Source: CAD feature listing. Evaluate the final solid. Frame: model axes, mm. Face numbers are marked on the shaded views. A direction names the side the tool comes from. Give positions to 0.01 mm unless a question says otherwise; leave off trailing zeros. Order: outer loops, then holes, each group sorted by start corner. A loop starts at its lowest first (then second) coordinate and runs counter-clockwise, first axis right, second up. Notation, with made-up numbers: (54, 66.25) - (76, 66.25) arc R14 ccw to (76, 75.25) - close; hole circle Ø7 at (-12.75, 42.5). An arc over 180 degrees is marked (long way). Answer as CSV lines item,"result".
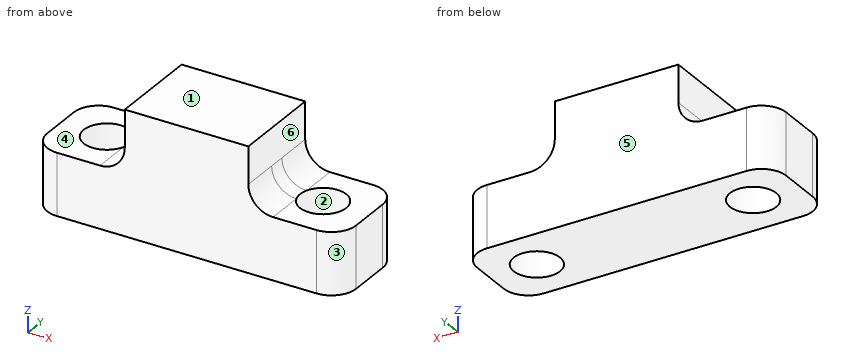
```python
from build123d import *

# Parameters (mm, degrees)
F1_DEPTH = 19.05
F3_DEPTH = 25.4
F4_R     = 5.08


with BuildPart() as f1:
    # F0 (on Front) → F1 (new body)
    with BuildSketch(Plane.XZ):
        Polygon((0, 12.7), (0, 0), (31.75, 0), (31.75, 25.4), (19.05, 25.4), (19.05, 12.7), align=None)
    extrude(amount=F1_DEPTH)

    # F2 (on face) → F3 (cut)
    with BuildSketch(Plane.XY.offset(12.7)):
        with BuildLine():
            ThreePointArc((14.2875, -9.525), (12.8925960454, -6.1574039546), (9.525, -4.7625))
            Line((9.525, -4.7625), (9.525, -9.525))
            Line((9.525, -9.525), (4.7625, -9.525))
            ThreePointArc((4.7625, -9.525), (9.525, -14.2875), (14.2875, -9.525))
        make_face()
        with BuildLine():
            Line((9.525, -9.525), (9.525, -4.7625))
            ThreePointArc((9.525, -4.7625), (6.1574039546, -6.1574039546), (4.7625, -9.525))
            Line((4.7625, -9.525), (9.525, -9.525))
        make_face()
    extrude(amount=-F3_DEPTH, mode=Mode.SUBTRACT)

    # F4
    f4_edges = [f1.edges().sort_by_distance(p)[0] for p in [
        (0, -19.05, 6.35),
        (0, 0, 6.35),
        (19.05, -9.525, 12.7),
    ]]
    fillet(f4_edges, radius=F4_R)

    # F5: F1 across face


with BuildPart() as f1_1:
    add(f1.part)
    add(f1.part.mirror(Plane(origin=(31.75, -9.525, 12.7), x_dir=(0, 1, 0), z_dir=(1, 0, 0))))


solid = f1_1.part
```
(1) Cut plane C-C (z = 6.5). Give the number of separate pieces and of enclosed holes in the cut face, then the cut area to 3 significant figures.
Completed:
separate pieces,"1"
enclosed holes,"2"
area,"1,050 mm²"
(2) Cut plane B-B (x = 51.5). Return loops of the section in (y, z), then the cut area to 3 significant figures.
Completed:
outline,"(-19.05, 0) - (-13.59, 0) - (-13.59, 12.7) - (-19.05, 12.7) - close; (-5.46, 0) - (0, 0) - (0, 12.7) - (-5.46, 12.7) - close"
area,"139 mm²"
(3) Contact query for flat-ended pins moving along their axis: pin 1 (4 mm diameter, centred on x = 5.5, y = -8.5, fed in from +Z); pin 2 (2.5 mm diameter, centred on y = -6.5, z = 23, fed in from -X); pin 3 (2.5 mm diameter, centred on y = -9, z = 19.5, fed in from +X). Output: stop coordinate, or through.
Completed:
pin 1,"z = 12.7"
pin 2,"x = 19.05"
pin 3,"x = 44.45"
(4) Mould query, pull axis Y, two halves, no side actions, for the marked faces 1, 2 and 3. Classes: released by +Y, released by -Y, zero draft, split by the parting line, or undercut.
Completed:
face 1,"zero draft"
face 2,"undercut"
face 3,"released by -Y"
(5) Cut plane D-D (y = -15.25). Return loops of the section in (x, z), then the cut area to 3 significant figures.
Completed:
outline,"(0.16, 0) - (63.34, 0) - (63.34, 12.7) - (49.53, 12.7) arc R5.08 cw to (44.45, 17.78) - (44.45, 25.4) - (19.05, 25.4) - (19.05, 17.78) arc R5.08 cw to (13.97, 12.7) - (0.16, 12.7) - close"
area,"1,140 mm²"
(6) Cut plane A-A (y = -12). Return loops of the section in (x, z).
Completed:
outline,"(0, 0) - (5.46, 0) - (5.46, 12.7) - (0, 12.7) - close; (13.59, 0) - (49.91, 0) - (49.91, 12.7) - (49.53, 12.7) arc R5.08 cw to (44.45, 17.78) - (44.45, 25.4) - (19.05, 25.4) - (19.05, 17.78) arc R5.08 cw to (13.97, 12.7) - (13.59, 12.7) - close; (58.04, 0) - (63.5, 0) - (63.5, 12.7) - (58.04, 12.7) - close"
(7) Access query for the marked faces 4, 5 and 6. Directions: +Z, -Z, +X, -X, +Y, -Y. A direction counts if a zero-diameter tool reaches every point of the face in a straight line with its end or side. Return the directions, or none.
Completed:
face 4,"+Z, -X, +Y, -Y"
face 5,"+Z, -Z, +X, -X, +Y"
face 6,"+Z, +X, +Y, -Y"
(8) Ray query, line 1 (X direction, y = -12, z = 5.5); line 2 (Z direction, x = 58.5, y = -5.5); line 3 (X direction, y = -2.25, z = 23.5). Return the intervals inside material, ascending. Write a range as from..to.
Completed:
line 1,"0..5.46, 13.59..49.91, 58.04..63.5"
line 2,"0..12.7"
line 3,"19.05..44.45"
